Input: part model. Units: mm. Frame: model coordinates. Face numbers are marked on the shaded views. Coordinates: 2 decimals unless noted, no trailing zeros. Write each loop counter-clockwise with the first axis right and the second up, starting at its lowest first coordinate (ties: lowest second). Pieces come first, ordered by that corner, then holes. Notation, with made-up numbers: (28, 33) - (39, 33) arc R14 ccw to (39, 49) - close; hole circle Ø6 at (26.25, 85.5). An arc over 180 degrees is marked (long way). Use CSV: the item, a comma, the result in double quotes.
```python
from build123d import *

# Parameters (mm, degrees)
SKETCH_1_W                   = 111
SKETCH_1_H                   = 77
SKETCH_1_R                   = 2
EXTRUDE_1_DEPTH              = 5
SKETCH_2_W                   = 108
SKETCH_2_H                   = 74
SKETCH_2_W_2                 = 94
SKETCH_2_H_2                 = 60
CUT_EXTRUDE_1_DEPTH          = 4.5
CUT_EXTRUDE_2_DEPTH          = 4
FILLET_1_R                   = 4
HOLE_WIZARD_M4_1_D           = 4.5
HOLE_WIZARD_M4_1_CSINK_D     = 9.4
HOLE_WIZARD_M4_1_CSINK_ANGLE = 90


with BuildPart() as part:
    # ｽｹｯﾁ1 → ﾎﾞｽ - 押し出し1 (new body)
    with BuildSketch(Plane.XY):
        with Locations((0, -6)):
            Rectangle(SKETCH_1_W, SKETCH_1_H)
        with Locations((-42, 19)):
            Circle(SKETCH_1_R, mode=Mode.SUBTRACT)
        with Locations(Location((42, 19, 0), (0, 0, 180))):
            Circle(SKETCH_1_R, mode=Mode.SUBTRACT)
        with Locations((42, -31)):
            Circle(SKETCH_1_R, mode=Mode.SUBTRACT)
        with Locations(Location((-42, -31, 0), (0, 0, 180))):
            Circle(SKETCH_1_R, mode=Mode.SUBTRACT)
    extrude(amount=EXTRUDE_1_DEPTH)

    # ｽｹｯﾁ2 → ｶｯﾄ - 押し出し1 (cut)
    with BuildSketch(Plane(origin=(0, 0, 0), x_dir=(-1, 0, 0), z_dir=(0, 0, -1))):
        with Locations((0, -6)):
            Rectangle(SKETCH_2_W, SKETCH_2_H)
        with Locations((0, -6)):
            Rectangle(SKETCH_2_W_2, SKETCH_2_H_2, mode=Mode.SUBTRACT)
    extrude(amount=-CUT_EXTRUDE_1_DEPTH, mode=Mode.SUBTRACT)

    # ｽｹｯﾁ3 → ｶｯﾄ - 押し出し2 (cut)
    with BuildSketch(Plane(origin=(0, 0, 0), x_dir=(-1, 0, 0), z_dir=(0, 0, -1))):
        with BuildLine():
            Line((-37, -31), (37, -31))
            ThreePointArc((37, -31), (38.464466094, -27.464466094), (42, -26))
            Line((42, -26), (42, 14))
            ThreePointArc((42, 14), (38.464466094, 15.464466094), (37, 19))
            Line((37, 19), (-37, 19))
            ThreePointArc((-37, 19), (-38.464466094, 15.464466094), (-42, 14))
            Line((-42, 14), (-42, -26))
            ThreePointArc((-42, -26), (-38.464466094, -27.464466094), (-37, -31))
        make_face()
    extrude(amount=-CUT_EXTRUDE_2_DEPTH, mode=Mode.SUBTRACT)

    # ﾌｨﾚｯﾄ1
    fillet_1_edges = [part.edges().sort_by_distance(p)[0] for p in [
        (-54, -43, 2.25),
        (54, -43, 2.25),
        (54, 31, 2.25),
        (-54, 31, 2.25),
        (47, -36, 2.25),
        (47, 24, 2.25),
        (-47, 24, 2.25),
        (-47, -36, 2.25),
        (-37, 19, 2),
        (-42, 14, 2),
        (-42, -26, 2),
        (-37, -31, 2),
        (37, -31, 2),
        (42, -26, 2),
        (42, 14, 2),
        (37, 19, 2),
        (-55.5, -44.5, 2.5),
        (-55.5, 32.5, 2.5),
        (55.5, 32.5, 2.5),
        (55.5, -44.5, 2.5),
    ]]
    fillet(fillet_1_edges, radius=FILLET_1_R)

    # M4 丸皿ねじ用皿穴1 (through all)
    with Locations(Plane.XY.offset(5)):
        with Locations((-42, 19), (-42, -31), (42, -31), (42, 19)):
            CounterSinkHole(HOLE_WIZARD_M4_1_D / 2, HOLE_WIZARD_M4_1_CSINK_D / 2, counter_sink_angle=HOLE_WIZARD_M4_1_CSINK_ANGLE)


solid = part.part
```
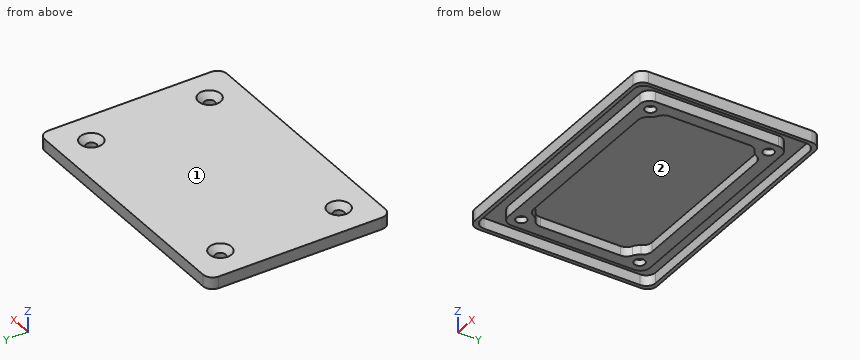
(1) Draft query along Y for the marked faces 1 and 2. Return one class per face: pulls with the +Y half, pulls with the -Y half, needs draft (parallel to the pull), parting line crosses it, or undercut.
Check values:
face 1,"needs draft"
face 2,"undercut"
(2) Cut plane A-A on z = 1.15. State how many separate pieces and enclosed holes the cut face has, and give its area (3 significant figures).
Check values:
separate pieces,"2"
enclosed holes,"6"
area,"2,010 mm^2"
(3) Cut plane B-B on x = 2.5. Return loops of the section in (y, z).
Check values:
outline,"(-44.5, 0) - (-43, 0) - (-43, 4.5) - (-36, 4.5) - (-36, 0) - (-31, 0) - (-31, 4) - (19, 4) - (19, 0) - (24, 0) - (24, 4.5) - (31, 4.5) - (31, 0) - (32.5, 0) - (32.5, 5) - (-44.5, 5) - close"
(4) Pin query (flat end, axial travel): pin 1 Ø2 at (x, y) = (-26.5, 13) entering from -Z. Return the tip coordinate at first contact, or that it passes through.
Check values:
pin 1,"z = 4"
(5) Ray query, probe 1 along X at (y, z) = (0, 1.75); probe 2 along Y at (x, z) = (-19.5, 1.4); probe 3 along Y at (x, z) = (-34.5, 4.4). Return the intervals inside material, ascending. Write a range as from..to.
Check values:
probe 1,"-55.5..-54, -47..-42, 42..47, 54..55.5"
probe 2,"-44.5..-43, -36..-31, 19..24, 31..32.5"
probe 3,"-44.5..-43, -36..24, 31..32.5"
(6) Cut plane C-C on y = -10. Return loops of the section in (x, z).
Check values:
outline,"(-55.5, 0) - (-54, 0) - (-54, 4.5) - (-47, 4.5) - (-47, 0) - (-42, 0) - (-42, 4) - (42, 4) - (42, 0) - (47, 0) - (47, 4.5) - (54, 4.5) - (54, 0) - (55.5, 0) - (55.5, 5) - (-55.5, 5) - close"
